Work out the finished part from the listing and answer in its coordinate system (mm). Face numbers are marked on the shaded views. A direction names the side the tool comes from. Round coordinates to 2 decimals unless told otherwise and drop trailing zeros. Loops run counter-clockwise (first coordinate to the right, second up) from the corner with the lowest first, then second, coordinate; pieces in that order, holes last. Notation, with made-up numbers: (-6.5, 80.5) -> (35.5, 80.5) arc R14 ccw to (35.5, 84.5) -> close; hole circle Ø9 at (40, -21). An arc over 180 degrees is marked (long way). Use one line per item in the form item = value.
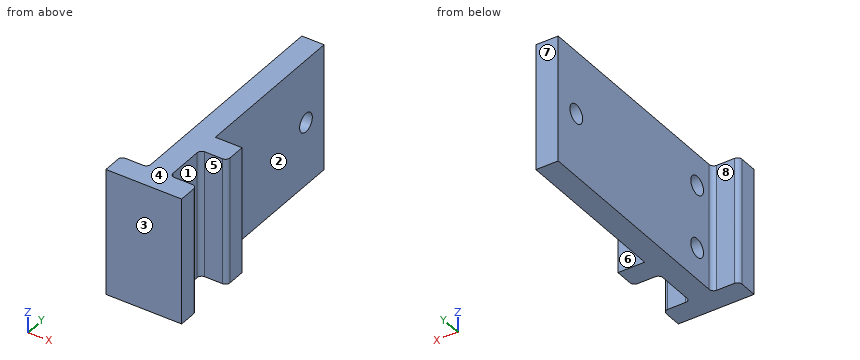
```python
from build123d import *

# Parameters (mm, degrees)
BOSS_EXTRUDE1_DEPTH = 56.8
CUT_EXTRUDE1_REACH  = 129.492
SKETCH2_R           = 4.2
CUT_EXTRUDE3_REACH  = 129.492
SKETCH4_R           = 4.2
FILLET1_R           = 2


with BuildPart() as part:
    # Sketch1 → Boss-Extrude1 (new body)
    with BuildSketch(Plane.XY):
        Polygon((0, 0), (0, 10), (12, 10), (12, 112), (22, 112), (22, 40), (34, 40), (34, 30), (22, 30), (22, 10), (34, 10), (34, 0), align=None)
    extrude(amount=BOSS_EXTRUDE1_DEPTH)

    # Sketch2 → Cut-Extrude1 (cut, up to next)
    with BuildSketch(Plane.ZY.offset(-12), mode=Mode.PRIVATE) as cut_extrude1_sk1:
        with Locations(Location((14.2, 20, 0), (0, 0, 270))):
            Circle(SKETCH2_R)
    cut_extrude1_tool1 = extrude(cut_extrude1_sk1.sketch, amount=-CUT_EXTRUDE1_REACH, mode=Mode.PRIVATE) & part.part
    # Sketch2 → Cut-Extrude1 (cut, up to next)
    with BuildSketch(Plane.ZY.offset(-12), mode=Mode.PRIVATE) as cut_extrude1_sk2:
        with Locations(Location((42.6, 20, 0), (0, 0, 270))):
            Circle(SKETCH2_R)
    cut_extrude1_tool2 = extrude(cut_extrude1_sk2.sketch, amount=-CUT_EXTRUDE1_REACH, mode=Mode.PRIVATE) & part.part
    add(cut_extrude1_tool1.solids().sort_by_distance((12, 20, 14.2))[0], mode=Mode.SUBTRACT)
    add(cut_extrude1_tool2.solids().sort_by_distance((12, 20, 42.6))[0], mode=Mode.SUBTRACT)

    # Sketch4 → Cut-Extrude3 (cut, up to next)
    with BuildSketch(Plane.ZY.offset(-12), mode=Mode.PRIVATE) as cut_extrude3_sk1:
        with Locations(Location((28.4, 100, 0), (0, 0, 270))):
            Circle(SKETCH4_R)
    cut_extrude3_tool1 = extrude(cut_extrude3_sk1.sketch, amount=-CUT_EXTRUDE3_REACH, mode=Mode.PRIVATE) & part.part
    add(cut_extrude3_tool1.solids().sort_by_distance((12, 100, 28.4))[0], mode=Mode.SUBTRACT)

    # Fillet1
    fillet1_edges = [part.edges().sort_by_distance(p)[0] for p in [
        (0, 10, 28.4),
        (12, 10, 28.4),
        (34, 30, 28.4),
        (22, 30, 28.4),
        (22, 10, 28.4),
        (34, 10, 28.4),
    ]]
    fillet(fillet1_edges, radius=FILLET1_R)


solid = part.part
```
(1) Find section A-A, the plane y = 100. Write down the section's boundary in (x, z), then the cut area to 3 significant figures.
Completed:
outline = (12, 0) -> (22, 0) -> (22, 24.2) -> (12, 24.2) -> close; (12, 32.6) -> (22, 32.6) -> (22, 56.8) -> (12, 56.8) -> close
area = 484 mm2
(2) Find section B-B, the plane z = 42.6. Write down the section's boundary in (x, y).
Completed:
outline = (0, 0) -> (34, 0) -> (34, 8) arc R2 ccw to (32, 10) -> (24, 10) arc R2 cw to (22, 12) -> (22, 15.8) -> (12, 15.8) -> (12, 12) arc R2 cw to (10, 10) -> (2, 10) arc R2 ccw to (0, 8) -> close; (12, 24.2) -> (22, 24.2) -> (22, 28) arc R2 cw to (24, 30) -> (32, 30) arc R2 ccw to (34, 32) -> (34, 40) -> (22, 40) -> (22, 112) -> (12, 112) -> close
(3) Consider L1, parallel to Z at x = 19.5, y = 20; L2, parallel to Y at x = 14, z = 14; L3, parallel to Y at x = 24.5, z = 21. Determine where each line is inside the solid, lowest interval first.
Completed:
L1 = 0 to 10, 18.4 to 38.4, 46.8 to 56.8
L2 = 0 to 15.8, 24.2 to 112
L3 = 0 to 10, 30 to 40
(4) Find section C-C, the plane x = 28. Write down the section's boundary in (y, z), then the cut area to 3 significant figures.
Completed:
outline = (0, 0) -> (10, 0) -> (10, 56.8) -> (0, 56.8) -> close; (30, 0) -> (40, 0) -> (40, 56.8) -> (30, 56.8) -> close
area = 1,140 mm2
(5) For the marked faces 4, 5, 6, 7 and 8, determine the directions among +Z, -Z, +X, -X, +Y, -Y from which every point of the face is accessible in a straight line to the end or side of a thin tool.
Completed:
face_4 = +Z, +X, -X, +Y, -Y
face_5 = +Z, -Z, +X
face_6 = +Z, -Z, +X, +Y
face_7 = +Z, -Z, +X, -X, +Y
face_8 = +Z, -Z, -X, +Y
(6) For a pull along Y with two mould halves and no side action, classify the marked faces 1, 2 and 3 as +Y half, -Y half, draft (parallel to the pull), parting line (faces both ways), or undercut.
Completed:
face_1 = undercut
face_2 = draft
face_3 = -Y half
(7) Given P1, Ø6.5, axis at x = 26, z = 39.5, coming from the +Y side; P2, Ø3, axis at y = 35, z = 43.5, coming from the -X side; P3, Ø10, axis at x = 3.5, y = 29, coming from the -Z side; P4, Ø1.5, axis at y = 54, z = 34.5, coming from the +X side, each flat-ended and moving along its own axis, determine where each tip first touches the part or whether it passes through.
Completed:
P1 = 40
P2 = 12
P3 = through
P4 = 22
(8) Find section D-D, the plane y = 20. Write down the section's boundary in (x, z).
Completed:
outline = (12, 0) -> (22, 0) -> (22, 10) -> (12, 10) -> close; (12, 18.4) -> (22, 18.4) -> (22, 38.4) -> (12, 38.4) -> close; (12, 46.8) -> (22, 46.8) -> (22, 56.8) -> (12, 56.8) -> close
